Drawing for the job (mm, zero at the part's lowest x, y, z). Round coordinates to 2 decimals unless told otherwise and drop trailing zeros. Write each loop counter-clockwise with the first axis right and the second up, starting at its lowest first coordinate (ties: lowest second). Pieces come first, ordered by that corner, then holes.
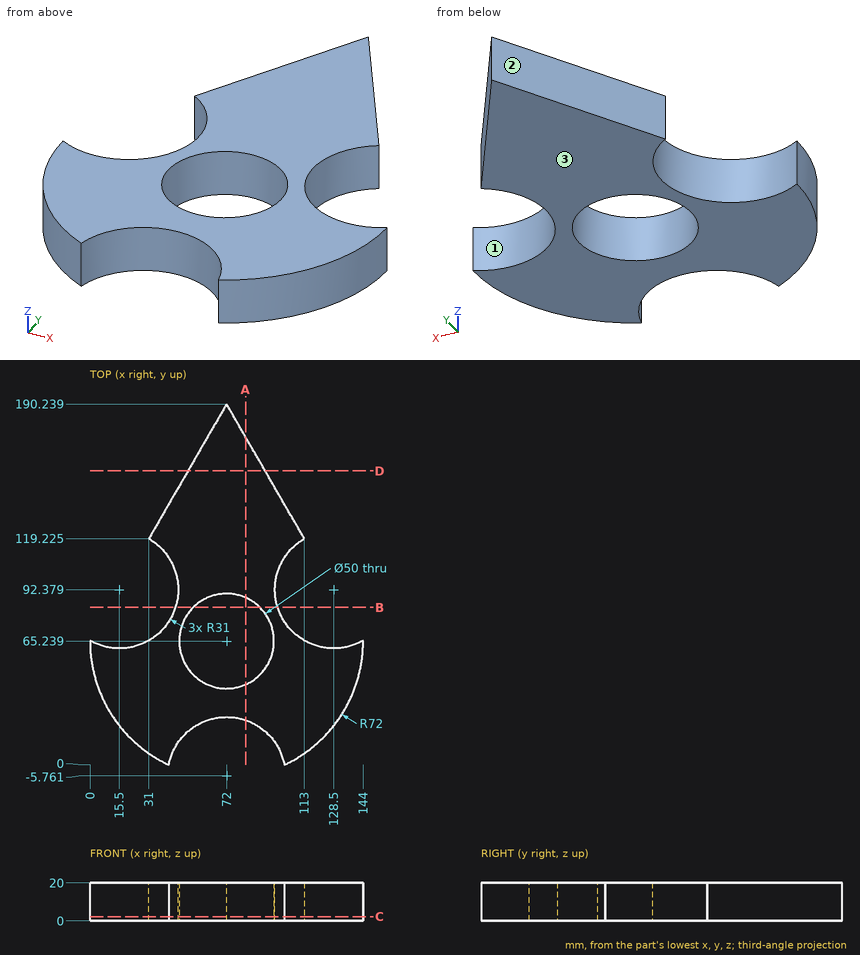
1) Pull direction Y, two halves, no side cores. Call the marked faces 1, 2 and 3: released by +Y, released by -Y, zero draft, split by the parting line, or undercut.
2) Cut at D-D on y = 155. List the corners of the cut face in (x, z) (1 decimal).
3) Wall check: probe 1 along Y at (x, z) = (72, 10.25); probe 2 along X at (y, z) = (66.5, 14.25) (1 decimal); probe 3 along Y at (x, z) = (87.5, 12.25) (1 decimal). Give the ranges that are in metal, low to high.
4) Cut at A-A on x = 82. List the corners of the cut face in (y, z), and give its area (3 significant figures).
5) Flat gauge pins, fed straight in: pin 1 Ø2 at (x, z) = (14.5, 10) entering from -Y; pin 2 Ø8 at (y, z) = (110, 16) entering from +X (1 decimal); pin 3 Ø10 at (x, z) = (92, 8.5) entering from -Y. Where does each tip first touch, or does it go through?
6) Cut at B-B on y = 83. List the corners of the cut face in (x, z) (1 decimal).
7) Cut at C-C on z = 2.25. List the corners of the cut face in (x, y) (1 decimal), and give its area (4 significant figures).
Result sheet:
1. face 1: undercut
1. face 2: released by +Y
1. face 3: zero draft
2. outline: (51.7, 0) - (92.3, 0) - (92.3, 20) - (51.7, 20) - close
3. probe 1: y = 25.24 to 40.24, 90.24 to 190.24
3. probe 2: x = 32.6 to 47, 97 to 111.4
3. probe 3: y = 21.1 to 45.6, 84.9 to 163.4
4. outline: (23.58, 0) - (42.33, 0) - (42.33, 20) - (23.58, 20) - close; (88.15, 0) - (172.92, 0) - (172.92, 20) - (88.15, 20) - close
4. area: 2,070 mm2
5. pin 1: stops at y = 20.61
5. pin 2: stops at x = 106.3
5. pin 3: stops at y = 12.57
6. outline: (45, 0) - (54.4, 0) - (54.4, 20) - (45, 20) - close; (89.6, 0) - (99, 0) - (99, 20) - (89.6, 20) - close
7. outline: (0, 65.5) arc R72 ccw to (41.5, 0) arc R31 cw to (102.5, 0) arc R72 ccw to (144, 65.5) arc R31 cw to (113, 119.2) - (72, 190.2) - (31, 119.2) arc R31 cw to start; hole circle Ø50 at (72, 65.2)
7. area: 10,750 mm2
